Check sheet for the modelled part. Datum: model origin and axes. Units: mm. Face numbers are marked on the shaded views. A direction names the side the tool comes from. Coordinates: 2 decimals unless noted, no trailing zeros. Loops run counter-clockwise (first coordinate to the right, second up) from the corner with the lowest first, then second, coordinate; pieces in that order, holes last. Notation, with made-up numbers: M 24,-39 L 51,-39 A19 cw 51,-35 Z; hole C -29,33.25 d3. An arc over 180 degrees is marked long. Use CSV: the item, a comma, the result in double quotes. Start each with the question number.
(1) Section check C-C on y = 434. Record the cut outline in (x, z).
(2) Section check A-A on z = 90. Record the cut outline in (x, y).
(3) Draft check along X on the marked faces 3, 4 and 5. Enter one of: pulls with the +X half, pulls with the -X half, needs draft (parallel to the pull), parting line crosses it, or undercut.
(4) Go/stop test with flat-tipped pins: pin 1 Ø2 at (y, z) = (187.5, 31.5) entering from -X; pin 2 Ø1.5 at (x, z) = (-38.5, 52) entering from +Y; pin 3 Ø3 at (x, z) = (-156.5, 62) entering from +Y. Record where each tip stops, or that it passes through.
(5) Scan lines: line 1 (X direction, y = 55, z = 61); line 2 (Z direction, x = -148, y = 308); line 3 (Y direction, x = 251, z = 121.5). Record each from-to range of solid material in increasing order.
(6) Section check D-D on x = 248. Record the cut outline in (y, z), and give its area (3 significant figures).
(7) Section check B-B on y = 197.5. Record the cut outline in (x, z).
(8) Set-up check for the marked faces 1 and 2: record each of +Z, -Z, +X, -X, +Y, -Y from which the full face is reachable in a straight line by a thin tool's end or side.
from build123d import *

# Parameters (mm, degrees)
BOSS_EXTRUDE1_DEPTH      = 12.7
BOSS_EXTRUDE2_DEPTH      = 152.3
BOSS_EXTRUDE2_DEPTH_BACK = 25
BOSS_EXTRUDE3_DEPTH      = 15.8
SKETCH4_W                = 12.7
SKETCH4_H                = 380
BOSS_EXTRUDE4_DEPTH      = 125


with BuildPart() as part:
    # Sketch1 → Boss-Extrude1 (new body)
    with BuildSketch(Plane.XY):
        with BuildLine():
            Line((320, 0.313790229), (-320, 0.313790229))
            Line((-320, 0.313790229), (-320, 393.313790229))
            Line((-320, 393.313790229), (-221.273103969, 450.313790229))
            ThreePointArc((-221.273103969, 450.313790229), (0, 332.5), (221.273103969, 450.313790229))
            Line((221.273103969, 450.313790229), (320, 393.313790229))
            Line((320, 393.313790229), (320, 0.313790229))
        make_face()
    extrude(amount=BOSS_EXTRUDE1_DEPTH)

    # Sketch2 → Boss-Extrude2 (add, two sides)
    with BuildSketch(Plane.XY.offset(12.7)) as boss_extrude2_sk:
        with BuildLine():
            Line((234.52055347, 472.2), (223.517731773, 478.552482069))
            ThreePointArc((223.517731773, 478.552482069), (0, 345.2), (-223.517731773, 478.552482069))
            Line((-223.517731773, 478.552482069), (-234.52055347, 472.2))
            ThreePointArc((-234.52055347, 472.2), (0, 332.5), (234.52055347, 472.2))
        make_face()
    extrude(amount=BOSS_EXTRUDE2_DEPTH)
    extrude(boss_extrude2_sk.sketch, amount=-BOSS_EXTRUDE2_DEPTH_BACK)

    # Sketch3 → Boss-Extrude3 (add)
    with BuildSketch(Plane.XZ.offset(-0.313790229)):
        Polygon((-305, -15), (305, -15), (320, 0), (320, 130), (305, 145), (-305, 145), (-320, 130), (-320, 0), align=None)
    extrude(amount=BOSS_EXTRUDE3_DEPTH)

    # Sketch4 → Boss-Extrude4 (add)
    with BuildSketch(Plane.XY.offset(12.7)):
        with Locations((-156.35, 190.313790229)):
            Rectangle(SKETCH4_W, SKETCH4_H)
        with Locations((156.35, 190.313790229)):
            Rectangle(SKETCH4_W, SKETCH4_H)
    extrude(amount=BOSS_EXTRUDE4_DEPTH)


solid = part.part
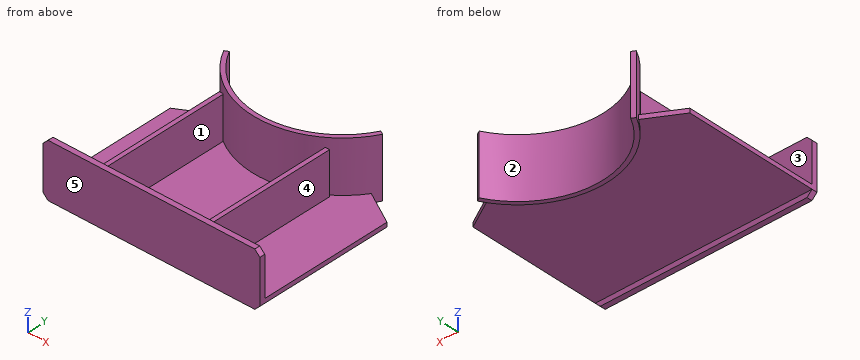
Outcome:
1,outline,"M -249.53,0 L -209.37,0 L -209.37,-12.3 L -192.94,-12.3 L -192.94,165 L -209.37,165 L -209.37,12.7 L -249.53,12.7 Z; M 192.94,-12.3 L 209.37,-12.3 L 209.37,0 L 249.53,0 L 249.53,12.7 L 209.37,12.7 L 209.37,165 L 192.94,165 Z"
2,outline,"M -320,-15.49 L 320,-15.49 L 320,0.31 L 162.7,0.31 L 162.7,380.31 L 152.37,380.31 A266.7 ccw 234.52,472.2 L 223.52,478.55 A254 cw -223.52,478.55 L -234.52,472.2 A266.7 ccw -152.37,380.31 L -162.7,380.31 L -162.7,0.31 L -320,0.31 Z; hole M -150,0.31 L 150,0.31 L 150,378.68 A266.7 cw -150,378.68 Z"
3,face 3,"undercut"
3,face 4,"pulls with the +X half"
3,face 5,"needs draft"
4,pin 1,"stops at x = -162.7"
4,pin 2,"stops at y = 348.25"
4,pin 3,"stops at y = 400.32"
5,line 1,"x = -162.7 to -150, 150 to 162.7"
5,line 2,"z = 0 to 12.7"
5,line 3,"y = -15.49 to 0.31"
6,outline,"M -15.49,-15 L 0.31,-15 L 0.31,0 L 434.88,0 L 434.88,12.7 L 0.31,12.7 L 0.31,145 L -15.49,145 Z"
6,area,"8,050 mm²"
7,outline,"M -320,0 L 320,0 L 320,12.7 L 162.7,12.7 L 162.7,137.7 L 150,137.7 L 150,12.7 L -150,12.7 L -150,137.7 L -162.7,137.7 L -162.7,12.7 L -320,12.7 Z"
8,face 1,"+Z"
8,face 2,"+Z, -Z, +Y"
